Autodesk Inventor part; units mm, degrees
ref_plane "YZ Plane" through (0, 0, 0) normal (1, 0, 0) x (0, 1, 0)
ref_plane "XZ Plane" through (0, 0, 0) normal (0, 1, 0) x (-1, 0, 0)
ref_plane "XY Plane" through (0, 0, 0) normal (0, 0, 1) x (1, 0, 0)
sketch "Sketch2" plane through (0, 0, 0) normal (0, 0, 1) x (1, 0, 0)
  line L0 (0, 0) -> (0, 20)
  line L1 (0, 20) -> (-85, 20)
  line L2 (-85, 20) -> (-85, 0)
  line L3 (-85, 0) -> (0, 0)
  line L4 (-85, 20) -> (-63.5526, 0)
  dimension "d10" = 20
  dimension "d30" = 85
  dimension "d31" = 43
extrude "Plate1" add sketch "Sketch2" along normal blind 2 contours L3 L4 L1 L0
fillet "Corner Round2" radius 10 1 edges at (0, 0, 1)
chamfer "Corner Chamfer1" distance 6 angle 45 1 edges at (-85, 20, 1)
equation "\"d7\" = Thickness"
equation "\"BendReliefWidth\" = Thickness"
equation "\"BendReliefDepth\" = 0.5 * Thickness"
equation "\"CornerReliefSize\" = 4 * Thickness"
equation "\"MinimumRemnant\" = 2 * Thickness"
equation "\"TransitionRadius\" = BendRadius"
equation "\"JacobiRadiusSize\" = BendRadius"
equation "\"GapSize\" = Thickness"
properties part number "MSC 125 ROСKET PILLAR" material "Stainless Steel"
The listing builds one solid part. Answer for the finished solid, in the listing's coordinates (mm). Coordinates: 2 decimals unless noted, no trailing zeros. Loops run counter-clockwise (first coordinate to the right, second up) from the corner with the lowest first, then second, coordinate; pieces in that order, holes last. Notation, with made-up numbers: M -15,31 L 35,31 A15 ccw 35,40 Z; hole C 54,2 d6. An arc over 180 degrees is marked long. Answer in a Markdown table with one row per item.
1) Find the intervals of material crossed by probe 1 along Y at (x, z) = (-76, 0.35); probe 2 along X at (y, z) = (8, 0.7); probe 3 along Y at (x, z) = (-67.5, 0.85), in increasing order.
Answers below:
| item | result |
|---|---|
| probe 1 | 11.61 to 20 |
| probe 2 | -72.13 to -0.2 |
| probe 3 | 3.68 to 20 |
2) Find section B-B (y = 13.25). Determine the outline of the cut face in (x, z).
Answers below:
| item | result |
|---|---|
| outline | M -77.76,0 L 0,0 L 0,2 L -77.76,2 Z |
3) Find section A-A (z = 0.6). Determine the outline of the cut face in (x, y), then the cut area to 3 significant figures.
Answers below:
| item | result |
|---|---|
| outline | M -80.61,15.91 L -63.55,0 L -10,0 A10 ccw 0,10 L 0,20 L -79,20 Z |
| area | 1,450 mm^2 |
4) Find section C-C (y = 8.75). Determine the outline of the cut face in (x, z), then the cut area to 3 significant figures.
Answers below:
| item | result |
|---|---|
| outline | M -72.94,0 L -0.08,0 L -0.08,2 L -72.94,2 Z |
| area | 146 mm^2 |
